from build123d import *

# Parameters (mm, degrees)
SKETCH2_R           = 3.15
SKETCH2_R_2         = 2.75
BOSS_EXTRUDE1_DEPTH = 2


with BuildPart() as part:
    # Sketch2 → Boss-Extrude1 (new body)
    with BuildSketch(Plane(origin=(0, 0, 0), x_dir=(1, 0, 0), z_dir=(0, 1, 0))):
        with BuildLine():
            Line((23.6, 5), (0, 5))
            ThreePointArc((0, 5), (-5, 0), (0, -5))
            Line((0, -5), (23.6, -5))
            ThreePointArc((23.6, -5), (28.6, 0), (23.6, 5))
        make_face()
        with Locations(Location((23.6, 0, 0), (0, 0, 270))):
            Circle(SKETCH2_R, mode=Mode.SUBTRACT)
        with Locations(Location((12.6, 0, 0), (0, 0, 90))):
            Circle(SKETCH2_R, mode=Mode.SUBTRACT)
        with Locations(Location((0, 0, 0), (0, 0, 270))):
            Circle(SKETCH2_R_2, mode=Mode.SUBTRACT)
    extrude(amount=-BOSS_EXTRUDE1_DEPTH)


solid = part.part
Here's how the part is built. I have some questions about the finished solid (model axes, mm). Round coordinates to 2 decimals unless told otherwise and drop trailing zeros. Loops run counter-clockwise (first coordinate to the right, second up) from the corner with the lowest first, then second, coordinate; pieces in that order, holes last.
1. If we section it at D-D on x = -1.5: Write out the boundary of the cut face in (y, z).
Answer list:
outline: (-2, -4.77) - (0, -4.77) - (0, -2.3) - (-2, -2.3) - close; (-2, 2.3) - (0, 2.3) - (0, 4.77) - (-2, 4.77) - close
2. If I drill on line 1 along X through (y, z) = (-1, 0); line 2 along Z through (x, y) = (12.6, -0.65); line 3 along X through (y, z) = (-0.1, 2), over which ranges is the centre line in solid material (lowest first)?
Answer list:
line 1: x = -5 to -2.75, 2.75 to 9.45, 15.75 to 20.45, 26.75 to 28.6
line 2: z = -5 to -3.15, 3.15 to 5
line 3: x = -4.58 to -1.89, 1.89 to 10.17, 15.03 to 21.17, 26.03 to 28.18
3. If we section it at B-B on y = -0.45: Write out the boundary of the cut face in (x, z), plus the area to 3 significant figures.
Answer list:
outline: (0, -5) - (23.6, -5) arc R5 ccw to (23.6, 5) - (0, 5) arc R5 ccw to start; hole circle Ø5.5 at (0, 0); hole circle Ø6.3 at (12.6, 0); hole circle Ø6.3 at (23.6, 0)
area: 228 mm2
4. For P1, Ø5.5, axis at x = 23.6, z = 0, coming from the +Y side, with a flat end and sliding along its axis, tell me the tip position at first contact or that it passes through.
Answer list:
P1: passes through
5. We'd pull the mould along X, two halves only. Please class faces 1 (the face through (-2.685, -0.986, -0.596)), 2 (the face through (-5, -1, 0)), 3 (the face through (28.6, -1, 0.1)): +X half, -X half, draft (parallel to the pull), parting line (faces both ways), or undercut.
Answer list:
face 1: undercut
face 2: -X half
face 3: +X half
6. If we section it at A-A on z = 0: Write out the boundary of the cut face in (x, y), plus the area to 3 significant figures.
Answer list:
outline: (-5, -2) - (-2.75, -2) - (-2.75, 0) - (-5, 0) - close; (2.75, -2) - (9.45, -2) - (9.45, 0) - (2.75, 0) - close; (15.75, -2) - (20.45, -2) - (20.45, 0) - (15.75, 0) - close; (26.75, -2) - (28.6, -2) - (28.6, 0) - (26.75, 0) - close
area: 31.0 mm2
7. If we section it at C-C on x = 12.6: Write out the boundary of the cut face in (y, z).
Answer list:
outline: (-2, -5) - (0, -5) - (0, -3.15) - (-2, -3.15) - close; (-2, 3.15) - (0, 3.15) - (0, 5) - (-2, 5) - close
